Source: CAD feature listing. Evaluate the final solid. Frame: model axes, mm. A direction names the side the tool comes from. Round coordinates to 2 decimals unless told otherwise and drop trailing zeros. Loops run counter-clockwise (first coordinate to the right, second up) from the corner with the lowest first, then second, coordinate; pieces in that order, holes last. Notation, with made-up numbers: (66.25, -21.5) -> (112.25, -21.5) arc R32 cw to (112.25, 17.5) -> close; hole circle Ø4 at (-10, 54.5). An arc over 180 degrees is marked (long way). Return JSON: item names as keys, results as strings. Group by question number.
```python
from build123d import *

# Parameters (mm, degrees)
SKETCH1_W           = 35
SKETCH1_H           = 35
BOSS_EXTRUDE1_DEPTH = 2.5
FILLET1_R           = 2.5
SKETCH2_R           = 15.4
BOSS_EXTRUDE2_DEPTH = 19.4
SKETCH3_R           = 12.8
BOSS_EXTRUDE3_DEPTH = 11
SKETCH4_R           = 13.4
CUT_EXTRUDE1_DEPTH  = 15
SKETCH5_R           = 1.75
BOSS_EXTRUDE4_DEPTH = 15
BOSS_EXTRUDE5_START = 10
SKETCH6_R           = 1.75
BOSS_EXTRUDE5_DEPTH = 10
SKETCH7_R           = 1.6
CUT_EXTRUDE2_DEPTH  = 35.128433893


with BuildPart() as part:
    # Sketch1 → Boss-Extrude1 (new body)
    with BuildSketch(Plane(origin=(0, 0, 0), x_dir=(1, 0, 0), z_dir=(0, 1, 0))):
        Rectangle(SKETCH1_W, SKETCH1_H)
    extrude(amount=BOSS_EXTRUDE1_DEPTH)

    # Fillet1
    fillet1_edges = [part.edges().sort_by_distance(p)[0] for p in [
        (17.5, 1.25, 17.5),
        (-17.5, 1.25, 17.5),
        (-17.5, 1.25, -17.5),
        (17.5, 1.25, -17.5),
    ]]
    fillet(fillet1_edges, radius=FILLET1_R)

    # Sketch2 → Boss-Extrude2 (add)
    with BuildSketch(Plane(origin=(0, 2.5, 0), x_dir=(1, 0, 0), z_dir=(0, 1, 0))):
        with Locations(Location((0, 0, 0), (0, 0, 90))):
            Circle(SKETCH2_R)
    extrude(amount=BOSS_EXTRUDE2_DEPTH)

    # Sketch3 → Boss-Extrude3 (add)
    with BuildSketch(Plane.XZ):
        with Locations(Location((0, 0, 0), (0, 0, 270))):
            Circle(SKETCH3_R)
    extrude(amount=BOSS_EXTRUDE3_DEPTH)

    # Sketch4 → Cut-Extrude1 (cut)
    with BuildSketch(Plane(origin=(0, 21.9, 0), x_dir=(1, 0, 0), z_dir=(0, 1, 0))):
        with Locations(Location((0, 0, 0), (0, 0, 270))):
            Circle(SKETCH4_R)
    extrude(amount=-CUT_EXTRUDE1_DEPTH, mode=Mode.SUBTRACT)

    # Sketch5 → Boss-Extrude4 (add)
    with BuildSketch(Plane(origin=(0, 6.9, 0), x_dir=(1, 0, 0), z_dir=(0, 1, 0))):
        with Locations(Location((-5, 5, 0), (0, 0, 270))):
            Circle(SKETCH5_R)
        with Locations(Location((-5, -5, 0), (0, 0, 270))):
            Circle(SKETCH5_R)
        with Locations(Location((5, -5, 0), (0, 0, 270))):
            Circle(SKETCH5_R)
        with Locations(Location((5, 5, 0), (0, 0, 270))):
            Circle(SKETCH5_R)
    extrude(amount=BOSS_EXTRUDE4_DEPTH)

    # Sketch6 → Boss-Extrude5 (add)
    with BuildSketch(Plane.XZ.offset(11).offset(BOSS_EXTRUDE5_START)):
        with Locations(Location((5, -5, 0), (0, 0, 90))):
            Circle(SKETCH6_R)
        with Locations(Location((5, 5, 0), (0, 0, 90))):
            Circle(SKETCH6_R)
        with Locations(Location((-5, 5, 0), (0, 0, 90))):
            Circle(SKETCH6_R)
        with Locations(Location((-5, -5, 0), (0, 0, 90))):
            Circle(SKETCH6_R)
    extrude(amount=-BOSS_EXTRUDE5_DEPTH)

    # Sketch7 → Cut-Extrude2 (cut, through all)
    with BuildSketch(Plane(origin=(0, 2.5, 0), x_dir=(1, 0, 0), z_dir=(0, 1, 0))):
        with Locations(Location((-13.5, 13.5, 0), (0, 0, 270))):
            Circle(SKETCH7_R)
        with Locations(Location((-13.5, -13.5, 0), (0, 0, 270))):
            Circle(SKETCH7_R)
        with Locations(Location((13.5, -13.5, 0), (0, 0, 270))):
            Circle(SKETCH7_R)
        with Locations(Location((13.5, 13.5, 0), (0, 0, 270))):
            Circle(SKETCH7_R)
    extrude(amount=-CUT_EXTRUDE2_DEPTH, mode=Mode.SUBTRACT)


solid = part.part
```
(1) Cut plane D-D (y = -1). Return loops of the section in (x, z).
(2) Set-up query: faces 1 (the face through (-12, 0, -8)), 2 (the face through (-13.43, 1.27, -15.1)), 3 (the face through (-16, 2.5, 0)). Return all of +Z, -Z, +X, -X, +Y, -Y with unobstructed straight access to the full face (end or side cutting, diameter ignored); none if empty.
(3) Mould query, pull axis Z, two halves, no side actions, for faces 4 (the face through (-3.29, -16.07, -5.38)), 5 (the face through (5, -21, 5)), 6 (the face through (16.787, 1.268, -16.748)). Classes: released by +Z, released by -Z, zero draft, split by the parting line, or undercut.
(4) Cut plane A-A (y = -17.5). Return loops of the section in (x, z).
(5) Pin query (flat end, axial travel): pin 1 (1.5 mm diameter, centred on y = 5, z = -4.5, fed in from -X); pin 2 (2 mm diameter, centred on y = 7.5, z = 3.5, fed in from +X); pin 3 (13 mm diameter, centred on x = 5, z = -3, fed in from -Y); pin 4 (3 mm diameter, centred on x = 0, z = 1.5, fed in from -Y). Return the tip coordinate at first contact, or that it passes through.
(6) Ray query, line 1 (X direction, y = 1.55, z = 13.5); line 2 (X direction, y = 1, z = -13); line 3 (Y direction, x = -2.5, z = -11.5). Return the intervals inside material, ascending.
(7) Cut plane B-B (z = 0). Return loops of the section in (x, y).
Answers follow:
{
 "1": {"outline": "circle Ø25.6 at (0, 0)"},
 "2": {"face 1": "-Y", "face 2": "+Y, -Y", "face 3": "+Y"},
 "3": {"face 4": "undercut", "face 5": "zero draft", "face 6": "released by -Z"},
 "4": {"outline": "circle Ø3.5 at (-5, -5); circle Ø3.5 at (-5, 5); circle Ø3.5 at (5, -5); circle Ø3.5 at (5, 5)"},
 "5": {"pin 1": "x = -14.94", "pin 2": "x = 15.2", "pin 3": "y = -21", "pin 4": "y = -11"},
 "6": {"line 1": "-17.5 to -15.1, -11.9 to 11.9, 15.1 to 17.5", "line 2": "-17.5 to -15.02, -11.98 to 11.98, 15.02 to 17.5", "line 3": "-11 to 6.9"},
 "7": {"outline": "(-17.5, 0) -> (-12.8, 0) -> (-12.8, -11) -> (12.8, -11) -> (12.8, 0) -> (17.5, 0) -> (17.5, 2.5) -> (15.4, 2.5) -> (15.4, 21.9) -> (13.4, 21.9) -> (13.4, 6.9) -> (-13.4, 6.9) -> (-13.4, 21.9) -> (-15.4, 21.9) -> (-15.4, 2.5) -> (-17.5, 2.5) -> close"}
}
